from build123d import *

# Parameters (mm, degrees)
SKETCH_1_W          = 9
SKETCH_1_H          = 9
EXTRUDE_1_DEPTH     = 56
SKETCH_2_W          = 7
SKETCH_2_H          = 7
CUT_EXTRUDE_1_DEPTH = 56
SKETCH_3_R          = 1.5
CUT_EXTRUDE_2_DEPTH = 56


with BuildPart() as part:
    # ｽｹｯﾁ1 → ﾎﾞｽ - 押し出し1 (new body)
    with BuildSketch(Plane.XY):
        Rectangle(SKETCH_1_W, SKETCH_1_H)
    extrude(amount=EXTRUDE_1_DEPTH)

    # ｽｹｯﾁ2 → ｶｯﾄ - 押し出し1 (cut)
    with BuildSketch(Plane.XY.offset(56)):
        Rectangle(SKETCH_2_W, SKETCH_2_H)
    extrude(amount=-CUT_EXTRUDE_1_DEPTH, mode=Mode.SUBTRACT)

    # ｽｹｯﾁ3 → ｶｯﾄ - 押し出し2 (cut)
    with BuildSketch(Plane(origin=(0, 4.5, 0), x_dir=(1, 0, 0), z_dir=(0, 1, 0))):
        with Locations((0, -3.5)):
            Circle(SKETCH_3_R)
        with Locations((0, -52.5)):
            Circle(SKETCH_3_R)
    extrude(amount=-CUT_EXTRUDE_2_DEPTH, mode=Mode.SUBTRACT)


solid = part.part
Part model, mm, in its own coordinate system. A direction names the side the tool comes from. Coordinates: 2 decimals unless noted, no trailing zeros. Loops run counter-clockwise (first coordinate to the right, second up) from the corner with the lowest first, then second, coordinate; pieces in that order, holes last. Notation, with made-up numbers: (-17, 28.5) - (11, 28.5) arc R14 cw to (11, 51.5) - close; hole circle Ø2 at (82, 7.5). An arc over 180 degrees is marked (long way). Write each question's results on one line, items separated by ' | '. Start each with the question number.
Q1. Two-plate mould, pull along X, no slides. Class faces 3 (the flat face through (0, 4.5, 28)), 4 (the flat face through (-4.5, 0, 28)), 5 (the cylindrical face through (0, -4, 2)), 6 (the cylindrical face through (0, 4, 54)): +X half, -X half, draft (parallel to the pull), parting line (faces both ways), or undercut.
Q2. Which spindle directions (+Z, -Z, +X, -X, +Y, -Y) get a long thin tool onto all of the face, cutting with end or side? Do faces 1 (the cylindrical face through (0, 4, 2)), 2 (the flat face through (0, 3.5, 28)). Say none if no direction does.
Q3. Slice it at D-D on x = -0.75. Give the cut face in (y, z), and give its area (3 significant figures).
Q4. Probe line 1 along Z through (x, y) = (0, -3.9); line 2 along X through (y, z) = (-3.8, 52.5); line 3 along X through (y, z) = (-1, 40). List the from-to ranges inside material, lowest first.
Q5. Slice it at B-B on x = 2.5. Give the cut face in (y, z).
Q6. Slice it at A-A on z = 3.5. Give the cut face in (x, y), and give its area (3 significant figures).
Answer:
1) face 3: draft | face 4: -X half | face 5: undercut | face 6: undercut
2) face 1: +Y, -Y | face 2: +Z, -Z
3) outline: (-4.5, 0) - (-3.5, 0) - (-3.5, 2.2) - (-4.5, 2.2) - close; (-4.5, 4.8) - (-3.5, 4.8) - (-3.5, 51.2) - (-4.5, 51.2) - close; (-4.5, 53.8) - (-3.5, 53.8) - (-3.5, 56) - (-4.5, 56) - close; (3.5, 0) - (4.5, 0) - (4.5, 2.2) - (3.5, 2.2) - close; (3.5, 4.8) - (4.5, 4.8) - (4.5, 51.2) - (3.5, 51.2) - close; (3.5, 53.8) - (4.5, 53.8) - (4.5, 56) - (3.5, 56) - close | area: 102 mm2
4) line 1: z = 0 to 2, 5 to 51, 54 to 56 | line 2: x = -4.5 to -1.5, 1.5 to 4.5 | line 3: x = -4.5 to -3.5, 3.5 to 4.5
5) outline: (-4.5, 0) - (-3.5, 0) - (-3.5, 56) - (-4.5, 56) - close; (3.5, 0) - (4.5, 0) - (4.5, 56) - (3.5, 56) - close
6) outline: (-4.5, -4.5) - (-1.5, -4.5) - (-1.5, -3.5) - (-3.5, -3.5) - (-3.5, 3.5) - (-1.5, 3.5) - (-1.5, 4.5) - (-4.5, 4.5) - close; (1.5, -4.5) - (4.5, -4.5) - (4.5, 4.5) - (1.5, 4.5) - (1.5, 3.5) - (3.5, 3.5) - (3.5, -3.5) - (1.5, -3.5) - close | area: 26.0 mm2
